The model under review builds one solid part; all positions refer to its coordinate system, in mm. A direction names the side the tool comes from. Coordinates: 2 decimals unless noted, no trailing zeros. Loops run counter-clockwise (first coordinate to the right, second up) from the corner with the lowest first, then second, coordinate; pieces in that order, holes last. Notation, with made-up numbers: M -4.5,22.25 L -0.5,22.25 A32 ccw -0.5,61.25 Z; hole C 66,-19 d10. An arc over 180 degrees is marked long. Write item = value, one per line. Start each with the question number.
Q1. Wall thickness on probe 1 along X at (y, z) = (-15, -10); probe 2 along Z at (x, y) = (27.5, -3); probe 3 along Y at (x, z) = (-5.5, -7.5): over which ranges is each line inside the solid? List them lowest first.
Q2. Mouldability with a two-part tool opening along X and no side actions: class faces 1 (the face through (0, 30, -10)), 2 (the face through (30, -1, 160)), 3 (the face through (1.5, -20.14, -5.23)) as released by +X, released by -X, zero draft, split by the parting line, or undercut.
Q3. We need section B-B on y = 0. Give the boundary of the cut face in (x, z), and give its area (3 significant figures).
Q4. We need section D-D on y = -13. Give the boundary of the cut face in (x, z).
Q5. For faces 4 (the face through (30, 1, -9)), 5 (the face through (0.6, 25.3, 150)), 6 (the face through (0, 40, 155)), 7 (the face through (0, -10, -10)), list the 3-axis set-ups (+Z, -Z, +X, -X, +Y, -Y) from which the entire face can be reached by the end or side of a thin tool; tool diameter is ignored.
Q6. We need section A-A on z = 160. Give the boundary of the cut face in (x, y), and give its area (3 significant figures).
Q7. We need section C-C on x = -11. Give the boundary of the cut face in (y, z).
Q8. Clearance check with flat-ended pins moving along their axes: pin 1 Ø4 at (x, z) = (-22.5, 145.5) entering from -Y; pin 2 Ø3 at (x, z) = (-13, 44) entering from +Y; pin 3 Ø8 at (x, z) = (-0.5, -12) entering from -Y; pin 4 Ø3 at (x, z) = (-10, 141) entering from -Y. State where each tip first meets the part, or that it passes through.
from build123d import *

# Parameters (mm, degrees)
SKETCH1_R            = 25
BOSS_EXTRUDE1_DEPTH  = 150
SKETCH2_W            = 60
SKETCH2_H            = 60
BOSS_EXTRUDE2_DEPTH  = 20
SKETCH3_W            = 60
SKETCH3_H            = 60
BOSS_EXTRUDE3_DEPTH  = 20
SKETCH4_R            = 5
CUT_EXTRUDE1_DEPTH   = 20
SKETCH5_R            = 5
BOSS_EXTRUDE4_DEPTH  = 20
CHAMFER1_SIZE        = 2
CHAMFER2_SIZE        = 2
SKETCH6_R            = 25
BOSS_EXTRUDE5_DEPTH  = 150
SKETCH7_W            = 60
SKETCH7_H            = 60
BOSS_EXTRUDE6_DEPTH  = 20
SKETCH8_W            = 60
SKETCH8_H            = 60
BOSS_EXTRUDE7_DEPTH  = 20
SKETCH9_R            = 5
CUT_EXTRUDE2_DEPTH   = 20
SKETCH10_R           = 5
BOSS_EXTRUDE8_DEPTH  = 20
CHAMFER3_SIZE        = 2
CHAMFER4_SIZE        = 2
SKETCH11_R           = 25
BOSS_EXTRUDE9_DEPTH  = 150
SKETCH12_W           = 60
SKETCH12_H           = 60
BOSS_EXTRUDE10_DEPTH = 20
SKETCH13_W           = 60
SKETCH13_H           = 60
BOSS_EXTRUDE11_DEPTH = 20
SKETCH14_R           = 5
CUT_EXTRUDE3_DEPTH   = 20
SKETCH15_R           = 5
BOSS_EXTRUDE12_DEPTH = 20
CHAMFER5_SIZE        = 2
CHAMFER6_SIZE        = 2


with BuildPart() as part:
    # Sketch1 → Boss-Extrude1 (new body)
    with BuildSketch(Plane.XY):
        Circle(SKETCH1_R)
    extrude(amount=BOSS_EXTRUDE1_DEPTH)

    # Sketch2 → Boss-Extrude2 (add)
    with BuildSketch(Plane.XY):
        Rectangle(SKETCH2_W, SKETCH2_H)
    extrude(amount=-BOSS_EXTRUDE2_DEPTH)

    # Sketch3 → Boss-Extrude3 (add)
    with BuildSketch(Plane.XY.offset(150)):
        Rectangle(SKETCH3_W, SKETCH3_H)
    extrude(amount=BOSS_EXTRUDE3_DEPTH)

    # Sketch4 → Cut-Extrude1 (cut)
    with BuildSketch(Plane(origin=(0, -30, 0), x_dir=(1, 0, 0), z_dir=(0, 1, 0))):
        with Locations(Location((0, 10, 0), (0, 0, 270))):
            Circle(SKETCH4_R)
    extrude(amount=CUT_EXTRUDE1_DEPTH, mode=Mode.SUBTRACT)

    # Sketch5 → Boss-Extrude4 (add)
    with BuildSketch(Plane(origin=(0, 30, 0), x_dir=(1, 0, 0), z_dir=(0, 1, 0))):
        with Locations(Location((0, -160, 0), (0, 0, 270))):
            Circle(SKETCH5_R)
    extrude(amount=BOSS_EXTRUDE4_DEPTH)

    # Chamfer1
    chamfer1_edges = [part.edges().sort_by_distance(p)[0] for p in [
        (30, 0, -20),
        (30, -30, -10),
        (-30, -30, -10),
        (-30, 30, -10),
    ]]
    chamfer(chamfer1_edges, length=CHAMFER1_SIZE)

    # Chamfer2
    chamfer2_edges = [part.edges().sort_by_distance(p)[0] for p in [
        (30, 30, 160),
        (-30, 30, 160),
        (0, -30, 150),
        (-30, 0, 170),
    ]]
    chamfer(chamfer2_edges, length=CHAMFER2_SIZE)

    # Sketch6 → Boss-Extrude5 (add)
    with BuildSketch(Plane.XY):
        Circle(SKETCH6_R)
    extrude(amount=BOSS_EXTRUDE5_DEPTH)

    # Sketch7 → Boss-Extrude6 (add)
    with BuildSketch(Plane.XY):
        Rectangle(SKETCH7_W, SKETCH7_H)
    extrude(amount=-BOSS_EXTRUDE6_DEPTH)

    # Sketch8 → Boss-Extrude7 (add)
    with BuildSketch(Plane.XY.offset(150)):
        Rectangle(SKETCH8_W, SKETCH8_H)
    extrude(amount=BOSS_EXTRUDE7_DEPTH)

    # Sketch9 → Cut-Extrude2 (cut)
    with BuildSketch(Plane(origin=(0, -30, 0), x_dir=(1, 0, 0), z_dir=(0, 1, 0))):
        with Locations(Location((0, 10, 0), (0, 0, 270))):
            Circle(SKETCH9_R)
    extrude(amount=CUT_EXTRUDE2_DEPTH, mode=Mode.SUBTRACT)

    # Sketch10 → Boss-Extrude8 (add)
    with BuildSketch(Plane(origin=(0, 30, 0), x_dir=(1, 0, 0), z_dir=(0, 1, 0))):
        with Locations(Location((0, -160, 0), (0, 0, 270))):
            Circle(SKETCH10_R)
    extrude(amount=BOSS_EXTRUDE8_DEPTH)

    # Chamfer3
    chamfer3_edges = [part.edges().sort_by_distance(p)[0] for p in [
        (-30, 0, 0),
        (-30, 0, -20),
        (0, -30, -20),
        (30, -30, -10),
        (30, 0, -20),
    ]]
    chamfer(chamfer3_edges, length=CHAMFER3_SIZE)

    # Chamfer4
    chamfer4_edges = [part.edges().sort_by_distance(p)[0] for p in [
        (0, -30, 150),
        (30, 30, 160),
        (0, 30, 170),
        (-30, 0, 150),
    ]]
    chamfer(chamfer4_edges, length=CHAMFER4_SIZE)

    # Sketch11 → Boss-Extrude9 (add)
    with BuildSketch(Plane.XY):
        Circle(SKETCH11_R)
    extrude(amount=BOSS_EXTRUDE9_DEPTH)

    # Sketch12 → Boss-Extrude10 (add)
    with BuildSketch(Plane.XY):
        Rectangle(SKETCH12_W, SKETCH12_H)
    extrude(amount=-BOSS_EXTRUDE10_DEPTH)

    # Sketch13 → Boss-Extrude11 (add)
    with BuildSketch(Plane.XY.offset(150)):
        Rectangle(SKETCH13_W, SKETCH13_H)
    extrude(amount=BOSS_EXTRUDE11_DEPTH)

    # Sketch14 → Cut-Extrude3 (cut)
    with BuildSketch(Plane(origin=(0, -30, 0), x_dir=(1, 0, 0), z_dir=(0, 1, 0))):
        with Locations(Location((0, 10, 0), (0, 0, 270))):
            Circle(SKETCH14_R)
    extrude(amount=CUT_EXTRUDE3_DEPTH, mode=Mode.SUBTRACT)

    # Sketch15 → Boss-Extrude12 (add)
    with BuildSketch(Plane(origin=(0, 30, 0), x_dir=(1, 0, 0), z_dir=(0, 1, 0))):
        with Locations(Location((0, -160, 0), (0, 0, 270))):
            Circle(SKETCH15_R)
    extrude(amount=BOSS_EXTRUDE12_DEPTH)

    # Chamfer5
    chamfer5_edges = [part.edges().sort_by_distance(p)[0] for p in [
        (-30, -30, -10),
        (0, 30, -20),
        (30, 0, -20),
        (30, -30, -10),
        (0, 30, 0),
    ]]
    chamfer(chamfer5_edges, length=CHAMFER5_SIZE)

    # Chamfer6
    chamfer6_edges = [part.edges().sort_by_distance(p)[0] for p in [
        (-30, 0, 170),
        (0, 30, 150),
        (30, 30, 160),
        (-30, 0, 150),
        (0, -30, 150),
    ]]
    chamfer(chamfer6_edges, length=CHAMFER6_SIZE)


solid = part.part
Returned:
q1.probe_1 = -30 to -5, 5 to 30
q1.probe_2 = -20 to 0, 150 to 170
q1.probe_3 = -30 to 30
q2.face_1 = zero draft
q2.face_2 = released by +X
q2.face_3 = undercut
q3.outline = M -30,-20 L 28,-20 L 30,-18 L 30,0 L 25,0 L 25,150 L 30,150 L 30,170 L -28,170 L -30,168 L -30,152 L -28,150 L -25,150 L -25,0 L -30,0 Z
q3.area = 9,890 mm^2
q4.outline = M -30,-20 L 28,-20 L 30,-18 L 30,0 L 21.35,0 L 21.35,150 L 30,150 L 30,170 L -28,170 L -30,168 L -30,152 L -28,150 L -21.35,150 L -21.35,0 L -30,0 Z; hole C 0,-10 d10
q5.face_4 = +Z, -Z, +X, +Y, -Y
q5.face_5 = none
q5.face_6 = +Y
q5.face_7 = -Y
q6.outline = M -30,-30 L 30,-30 L 30,28 L 28,30 L 5,30 L 5,50 L -5,50 L -5,30 L -30,30 Z
q6.area = 3,800 mm^2
q7.outline = M -30,-20 L 28,-20 L 30,-18 L 30,-2 L 28,0 L 22.45,0 L 22.45,150 L 28,150 L 30,152 L 30,170 L -30,170 L -30,152 L -28,150 L -22.45,150 L -22.45,0 L -30,0 Z
q8.pin_1 = -14.31
q8.pin_2 = 22.2
q8.pin_3 = -30
q8.pin_4 = -23.51
